Input: part model. Units: mm. Frame: model coordinates. A direction names the side the tool comes from. Coordinates: 2 decimals unless noted, no trailing zeros. Order: outer loops, then holes, each group sorted by start corner. A loop starts at its lowest first (then second) coordinate and runs counter-clockwise, first axis right, second up. Notation, with made-up numbers: (61.25, -5.75) - (68.25, -5.75) arc R15 ccw to (68.25, 9.25) - close; hole circle Ø5 at (70, 89.5). An arc over 180 degrees is marked (long way). One line per question, with ' | ' between items. Start each with the question number.
Autodesk Inventor part; units mm, degrees
ref_plane "YZ Plane" through (0, 0, 0) normal (1, 0, 0) x (0, 1, 0)
ref_plane "XZ Plane" through (0, 0, 0) normal (0, 1, 0) x (-1, 0, 0)
ref_plane "XY Plane" through (0, 0, 0) normal (0, 0, 1) x (1, 0, 0)
sketch "Sketch1" plane through (0, 0, 0) normal (0, 1, 0) x (-1, 0, 0)
  line L0 (0, 0) -> (-190, 0)
  line L1 (0, 15) -> (0, 0)
  line L2 (-95, 0) -> (-95, 180)
  line L3 (0, 0) -> (0, 90)
  line L4 (-190, 0) -> (-190, 90)
  line L5 (-95, 180) -> (-75, 180)
  line L6 (-75, 180) -> (0, 90)
  line L7 (-95, 180) -> (-115, 180)
  line L8 (-115, 180) -> (-190, 90)
  dimension "d1" = 190
  dimension "d37" = 180
  dimension "d39" = 20
  dimension "d40" = 20
extrude "Extrusion1" add sketch "Sketch1" along normal blind 4
sketch "Sketch5" plane through (0, 4, 0) normal (0, 1, 0) x (1, 0, 0)
  circle A0 centre (27.5, -12) radius 1.55
  circle A1 centre (27.5, -43) radius 1.55
  circle A2 centre (162.5, -43) radius 1.55
  circle A3 centre (162.5, -12) radius 1.55
  point P0 (0, 0)
extrude "Extrusion2" cut sketch "Sketch5" against normal blind 10
sketch "Sketch6" plane through (0, 4, 0) normal (0, 1, 0) x (1, 0, 0)
  line L0 (64, -39.65) -> (64, -15.35)
  line L1 (190, 0) -> (0, 0)
  circle A0 centre (27.5, -43) radius 1.55
  circle A1 centre (27.5, -12) radius 1.55
  line L2 (64, -27.5) -> (64, -15.35)
  line L3 (64, -15.35) -> (70, -15.35)
  line L4 (70, -15.35) -> (70, -39.65)
  line L5 (70, -39.65) -> (64, -39.65)
  line L6 (190, 0) -> (0, 0)
  line L7 (126, -39.65) -> (126, -15.35)
  line L8 (126, -15.35) -> (120, -15.35)
  line L9 (120, -15.35) -> (120, -39.65)
  line L10 (120, -39.65) -> (126, -39.65)
  dimension "d131" = 6
  dimension "d132" = 6
extrude "Extrusion3" add sketch "Sketch6" along normal blind 5 contours L0 L3 L4 L5 | L10 L9 L8 L7
sketch "Sketch14" plane through (0, 4, 0) normal (0, 1, 0) x (1, 0, 0)
  line L0 (190, 0) -> (0, 0)
  line L1 (0, 0) -> (0, -7.5)
  line L2 (0, 0) -> (0, -15)
  line L3 (0, -90) -> (75, -180)
  circle A0 centre (7.5, -7.5) radius 1.55
  circle A1 centre (7.5, -90) radius 1.55
  line L4 (75, -180) -> (115, -180)
  circle A2 centre (182.5, -7.5) radius 1.55
  circle A3 centre (182.5, -90) radius 1.55
  circle A4 centre (95, -172.5) radius 1.55
  dimension "d68" = 7.5
  dimension "d71" = 3.1
  dimension "d72" = 3.1
  dimension "d74" = 3.1
extrude "Extrusion10" cut sketch "Sketch14" against normal blind 10
sketch "Sketch17" plane through (0, 4, 0) normal (0, 1, 0) x (1, 0, 0)
  circle A0 centre (95, -152.3364) radius 14.25
  line L0 (75, -180) -> (115, -180)
  point P0 (0, 0)
  dimension "d101" = 28.5
  dimension "d112" = 27.6636
extrude "Extrusion13" cut sketch "Sketch17" against normal through all
sketch "Sketch19" plane through (0, 4, 0) normal (0, 1, 0) x (1, 0, 0)
  circle A0 centre (95, -152.3364) radius 14.25
  circle A1 centre (114.5, -152.3364) radius 1.55
  circle A2 centre (75.5, -152.3364) radius 1.55
  point P0 (0, 0)
  dimension "d108" = 3.1
  dimension "d109" = 3.1
extrude "Extrusion14" cut sketch "Sketch19" against normal blind 5 contours A1 | A2
sketch "Sketch27" plane through (126, 4, 39.65) normal (1, 0, 0) x (0, 0, -1)
  circle A0 centre (12.15, 14.9) radius 2
  circle A1 centre (12.15, 14.9) radius 12.15
  arc A2 (5.1064, 5) -> (19.1936, 5) centre (12.15, 14.9) ccw
  line L0 (0, 5) -> (24.3, 5)
  line L1 (5.1064, 5) -> (19.1936, 5)
  point P0 (39.65, -4)
  point P1 (5.1064, 5)
extrude "Extrusion18" cut sketch "Sketch27" against normal through all contours L0 A1 picked at (10.6816, 4.5256)
sketch "Sketch28" plane through (0, 4, 0) normal (0, 1, 0) x (1, 0, 0)
  circle A0 centre (67, -44.8593) radius 1.5
  circle A1 centre (123, -44.8593) radius 1.5
  circle A2 centre (123.1217, -10.1201) radius 1.5
  circle A3 centre (67.1217, -10.1201) radius 1.5
  circle A4 centre (67.1217, -10.1201) radius 1.55
  circle A5 centre (123.1217, -10.1201) radius 1.55
  circle A6 centre (123, -44.8593) radius 1.55
  circle A7 centre (67, -44.8593) radius 1.55
  point P0 (0, 0)
  dimension "d135" = 3.1
  dimension "d136" = 3.1
  dimension "d137" = 3.1
  dimension "d138" = 3.1
extrude "Extrusion19" cut sketch "Sketch28" against normal blind 10 contours A0 | A1 | A2 | A3
sketch "Sketch29" plane through (0, 4, 0) normal (0, 1, 0) x (1, 0, 0)
  circle A0 centre (7.5, -7.5) radius 1.55
  circle A1 centre (182.5, -7.5) radius 1.55
  circle A2 centre (100, -7.5) radius 1.55
  line L0 (0, 0) -> (0, -90)
  dimension "d141" = 3.1
  dimension "d194" = 100
extrude "Extrusion20" cut sketch "Sketch29" against normal blind 10 contours A2
sketch "Sketch30" plane through (0, 4, 0) normal (0, 1, 0) x (1, 0, 0)
  circle A0 centre (100, -7.5) radius 1.55
  line L0 (120.6, -60.7864) -> (120.6, -133.0864)
  line L1 (69.4, -60.7864) -> (69.4, -133.0864)
  circle A1 centre (95, -152.3364) radius 14.25
  line L2 (120.6, -133.0864) -> (69.4, -133.0864)
  line L3 (120.6, -60.7864) -> (69.4, -60.7864)
  line L4 (69.4, -60.7864) -> (69.4, -133.0864)
  line L5 (120.6, -60.7864) -> (120.6, -133.0864)
  line L6 (69.4, -129.6517) -> (69.4, -60.7864)
  line L7 (120.6, -60.7864) -> (123, -60.7864)
  line L8 (123, -60.7864) -> (123, -133.0864)
  line L9 (123, -133.0864) -> (120.6, -133.0864)
  line L10 (120.6, -133.0864) -> (120.6, -60.7864)
  line L11 (69.4, -60.7864) -> (69.4, -133.0864)
  line L12 (69.4, -133.0864) -> (67, -133.0864)
  line L13 (67, -133.0864) -> (67, -60.7864)
  line L14 (67, -60.7864) -> (69.4, -60.7864)
  point P0 (0, 0)
  dimension "d148" = 51.2
  dimension "d149" = 72.3
  dimension "d151" = 2.4
  dimension "d152" = 2.4
extrude "Extrusion21" add sketch "Sketch30" along normal blind 5 contours L7 L8 L9 L0 | L1 L12 L13 L14
sketch "Sketch31" plane through (0, 4, 0) normal (0, 1, 0) x (1, 0, 0)
  line L0 (123, -60.7864) -> (123, -133.0864)
  line L1 (128, -73.8364) -> (160, -73.8364)
  line L2 (160, -73.8364) -> (160, -120.0364)
  line L3 (160, -120.0364) -> (128, -120.0364)
  line L4 (128, -120.0364) -> (128, -73.8364)
  line L5 (144, -73.8364) -> (144, -70.8364)
  line L6 (144, -120.0364) -> (144, -123.0364)
  circle A0 centre (144, -70.8364) radius 1
  circle A1 centre (144, -123.0364) radius 1
  point P0 (0, 0)
  dimension "d156" = 32
  dimension "d157" = 46.2
  dimension "d158" = 5
  dimension "d159" = 3
  dimension "d160" = 3
  dimension "d161" = 2
  dimension "d162" = 2
extrude "Extrusion22" cut sketch "Sketch31" against normal blind 2 contours A0 | A1
sketch "Sketch33" plane through (190, 0, 90) normal (0.7682, 0, 0.6402) x (0.6402, 0, -0.7682)
  line L0 (-117.1537, 0) -> (-117.1537, 4)
  line L1 (-117.1537, 4) -> (-82.1537, 4)
  line L2 (-117.1537, 4) -> (0, 4)
  line L3 (-82.1537, 4) -> (-82.1537, 12.45)
  line L4 (-82.1537, 12.45) -> (-67.6537, 12.45)
  line L5 (-67.6537, 12.45) -> (-67.6537, 4)
  line L6 (-82.1537, 4) -> (-87.1537, 4)
  line L7 (-87.1537, 4) -> (-87.1537, 16)
  line L8 (-87.1537, 16) -> (-62.6537, 16)
  line L9 (-62.6537, 16) -> (-62.6537, 4)
  point P0 (-52.4951, 0)
  dimension "d171" = 35
  dimension "d172" = 8.45
  dimension "d173" = 14.5
  dimension "d174" = 5
  dimension "d175" = 12
  dimension "d176" = 24.5
extrude "Extrusion24" add sketch "Sketch33" against normal blind 9 contours L7 L8 L9 L2 L5 L4 L3 L1
fillet "Fillet1" radius 2 1 edges at (130.7485, 4, 154.0725)
fillet "Fillet2" radius 2 1 edges at (146.4331, 4, 135.2511)
sketch "Sketch34" plane through (0, 4, 0) normal (0, 1, 0) x (1, 0, 0)
  line L0 (85, -79.4364) -> (105, -79.4364)
  line L1 (105, -79.4364) -> (105, -114.4364)
  line L2 (105, -114.4364) -> (85, -114.4364)
  line L3 (69.4, -60.7864) -> (69.4, -133.0864)
  line L4 (120.6, -60.7864) -> (120.6, -133.0864)
  line L5 (85, -79.4364) -> (85, -114.4364)
  point P0 (0, 0)
  dimension "d181" = 20
  dimension "d182" = 35
extrude "Extrusion25" cut sketch "Sketch34" against normal blind 10
fillet "Fillet3" radius 10 1 edges at (85, 2, 79.4364)
fillet "Fillet4" radius 10 3 edges at (105, 2, 114.4364) (105, 2, 79.4364) (85, 2, 114.4364)
sketch "Sketch35" plane through (0, 4, 0) normal (0, 1, 0) x (1, 0, 0)
  circle A0 centre (116.6, -54.3864) radius 1.5
  circle A1 centre (73.4, -54.3864) radius 1.5
  circle A2 centre (73.4, -139.4864) radius 1.5
  circle A3 centre (116.6, -139.4864) radius 1.5
  circle A4 centre (73.4, -54.3864) radius 1.55
  circle A5 centre (116.6, -54.3864) radius 1.55
  circle A6 centre (116.6, -139.4864) radius 1.55
  circle A7 centre (73.4, -139.4864) radius 1.55
  point P0 (0, 0)
  dimension "d188" = 3.1
  dimension "d189" = 3.1
  dimension "d190" = 3.1
  dimension "d191" = 3.1
extrude "Extrusion26" cut sketch "Sketch35" against normal through all contours A0 | A1 | A2 | A3
properties part number "bp_v3" material "PET Plastic"
(1) Section A-A (z = 98). Output: boundary loops of the cut face in (x, y).
(2) Section B-B (x = 154). Output: boundary loops of the cut face in (y, z).
(3) Reachability of faces 1 (the face through (70, 6, 27)), 2 (the face through (67, 6, 39.65)), 3 (the face through (146.48, 11.07, 135.29)), 4 (the face through (105, 2, 97)) from +Z, -Z, +X, -X, +Y, -Y: full face, straight path, thin tool, end or side. Return the list, or none.
(4) Pin query (flat end, axial travel): pin 1 (1.5 mm diameter, centred on y = 8.5, z = 66, fed in from -X); pin 2 (4 mm diameter, centred on x = 182.5, z = 7.5, fed in from +Y); pin 3 (1.5 mm diameter, centred on x = 122.5, y = 7.5, fed in from +Z); pin 4 (5 mm diameter, centred on y = 13.5, z = 114.5, fed in from -X). Return the tip coordinate at first contact, or that it passes through.
(5) Draft query along X for faces 5 (the face through (141.92, 12.75, 147.69)), 6 (the face through (123, 6, 15.35)), 7 (the face through (69.4, 6, 96)). Return one class per face: +X half, -X half, draft (parallel to the pull), parting line (faces both ways), or undercut.
(6) Section C-C (x = 14). Output: boundary loops of the cut face in (y, z), then the cut area to 3 significant figures.
(7) Material intervals for line 1 along Z through (x, y) = (95, 2.05); line 2 along X through (y, z) = (1.1, 90); line 3 along Z through (x, y) = (69.5, 5), sorted ascending. Write a range as from..to.
Worked answers:
1) outline: (6.67, 0) - (85, 0) - (85, 4) - (69.4, 4) - (69.4, 9) - (67, 9) - (67, 4) - (6.67, 4) - close; (105, 0) - (183.33, 0) - (183.33, 4) - (123, 4) - (123, 9) - (120.6, 9) - (120.6, 4) - (105, 4) - close
2) outline: (0, 0) - (4, 0) - (4, 133.2) - (0, 133.2) - close
3) face 1: +Z, -Z, +Y | face 2: +X, -X, +Y | face 3: -Z, +X, +Y | face 4: +Y, -Y
4) pin 1: stops at x = 67 | pin 2: stops at y = 4 | pin 3: stops at z = 133.09 | pin 4: passes through
5) face 5: +X half | face 6: draft | face 7: undercut
6) outline: (0, 0) - (4, 0) - (4, 106.8) - (0, 106.8) - close | area: 427 mm²
7) line 1: z = 0..79.44, 114.44..138.09, 166.59..170.95, 174.05..180 | line 2: x = 0..5.95, 9.05..85, 105..180.95, 184.05..190 | line 3: z = 15.35..39.65
